from build123d import *

# Parameters (mm, degrees)
F1_DEPTH       = 15
F2_R           = 3
F3_W           = 103
F3_H           = 8
F4_DEPTH       = 12
F5_W           = 103
F5_H           = 3
F6_DEPTH       = 3
F8_D           = 5
F8_CSINK_D     = 8
F8_CSINK_ANGLE = 90


with BuildPart() as f1:
    # F0 (on Top) → F1 (new body)
    with BuildSketch(Plane.XY):
        with BuildLine():
            Line((-67, -20), (67, -20))
            ThreePointArc((67, -20), (69.1213203436, -19.1213203436), (70, -17))
            Line((70, -17), (70, 7))
            ThreePointArc((70, 7), (69.1213203436, 9.1213203436), (67, 10))
            Line((67, 10), (-67, 10))
            ThreePointArc((-67, 10), (-69.1213203436, 9.1213203436), (-70, 7))
            Line((-70, 7), (-70, -17))
            ThreePointArc((-70, -17), (-69.1213203436, -19.1213203436), (-67, -20))
        make_face()
    extrude(amount=F1_DEPTH)

    # F2
    f2_edges = [f1.edges().sort_by_distance(p)[0] for p in [
        (0, -20, 0),
        (69.12132, -19.12132, 0),
        (70, -5, 0),
        (69.12132, 9.12132, 0),
        (0, 10, 0),
        (-69.12132, 9.12132, 0),
        (-70, -5, 0),
        (-69.12132, -19.12132, 0),
    ]]
    fillet(f2_edges, radius=F2_R)

    # F3 (on face) → F4 (cut)
    with BuildSketch(Plane.XY.offset(15)):
        Rectangle(F3_W, F3_H)
    extrude(amount=-F4_DEPTH, mode=Mode.SUBTRACT)

    # F5 (on face) → F6 (cut)
    with BuildSketch(Plane(origin=(0, 0, 0), x_dir=(1, 0, 0), z_dir=(0, 0, -1))):
        with Locations((0, 3.5)):
            Rectangle(F5_W, F5_H)
        with Locations((0, -3.5)):
            Rectangle(F5_W, F5_H)
    extrude(amount=-F6_DEPTH, mode=Mode.SUBTRACT)

    # F8 (through all)
    with Locations(Plane(origin=(0, 0, 0), x_dir=(1, 0, 0), z_dir=(0, 0, -1))):
        with Locations((-60, 5), (60, 5)):
            CounterSinkHole(F8_D / 2, F8_CSINK_D / 2, counter_sink_angle=F8_CSINK_ANGLE)


solid = f1.part
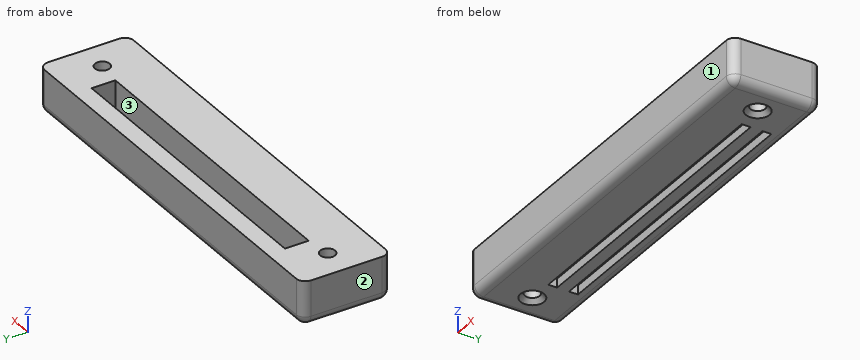
Part model, mm, in its own coordinate system. Face numbers are marked on the shaded views. Round coordinates to 2 decimals unless told otherwise and drop trailing zeros. Write each loop counter-clockwise with the first axis right and the second up, starting at its lowest first coordinate (ties: lowest second). Pieces come first, ordered by that corner, then holes. Notation, with made-up numbers: M 32.5,58.5 L 76.5,58.5 A10 ccw 76.5,69.5 Z; hole C 0.25,-34.5 d9. An arc over 180 degrees is marked long. Return JSON: item names as keys, results as strings. Group by question number.
(1) Saw through at C-C on x = -60. Write the cut outline in (y, z), then the cut area to 3 significant figures.
(2) Saw through at B-B on z = 5.75. Write the cut outline in (x, y), then the cut area to 3 significant figures.
(3) Saw through at A-A on x = 4.5. Write the cut outline in (y, z).
(4) Drill centre lines: probe 1 along Y at (x, z) = (4.5, 2.75); probe 2 along Y at (x, z) = (-60, 11.25); probe 3 along Y at (x, z) = (46, 12). Where is each one in solid material? Low to high.
(5) Pin check, flat tips, straight feed: pin 1 Ø1 at (x, z) = (-12.5, 2.5) entering from -Y; pin 2 Ø0.8 at (x, y) = (-10, 4.5) entering from -Z; pin 3 Ø0.9 at (x, z) = (-5, 1.5) entering from -Y; pin 4 Ø1.5 at (x, z) = (13, 1) entering from +Y. Stop position of each tip, or through.
(6) Two-plate mould, pull along Y, no slides. Class the marked faces 1, 2 and 3: +Y half, -Y half, draft (parallel to the pull), parting line (faces both ways), or undercut.
Returned:
{
 "1": {"outline": "M -20,3 A3 ccw -17,0 L -9,0 L -7.5,1.5 L -7.5,15 L -20,15 Z; M -2.5,1.5 L -1,0 L 7,0 A3 ccw 10,3 L 10,15 L -2.5,15 Z", "area": "369 mm²"},
 "2": {"outline": "M -70,-17 A3 ccw -67,-20 L 67,-20 A3 ccw 70,-17 L 70,7 A3 ccw 67,10 L -67,10 A3 ccw -70,7 Z; hole C -60,-5 d5; hole M -51.5,-4 L 51.5,-4 L 51.5,4 L -51.5,4 Z; hole C 60,-5 d5", "area": "3,330 mm²"},
 "3": {"outline": "M -20,3 A3 ccw -17,0 L -5,0 L -5,3 L -4,3 L -4,15 L -20,15 Z; M -2,0 L 2,0 L 2,3 L -2,3 Z; M 4,3 L 5,3 L 5,0 L 7,0 A3 ccw 10,3 L 10,15 L 4,15 Z"},
 "4": {"probe 1": "-19.99 to -5, -2 to 2, 5 to 9.99", "probe 2": "-20 to -7.5, -2.5 to 10", "probe 3": "-20 to -4, 4 to 10"},
 "5": {"pin 1": "y = -20", "pin 2": "z = 3", "pin 3": "y = -19.81", "pin 4": "y = 9.73"},
 "6": {"face 1": "-Y half", "face 2": "draft", "face 3": "undercut"}
}
